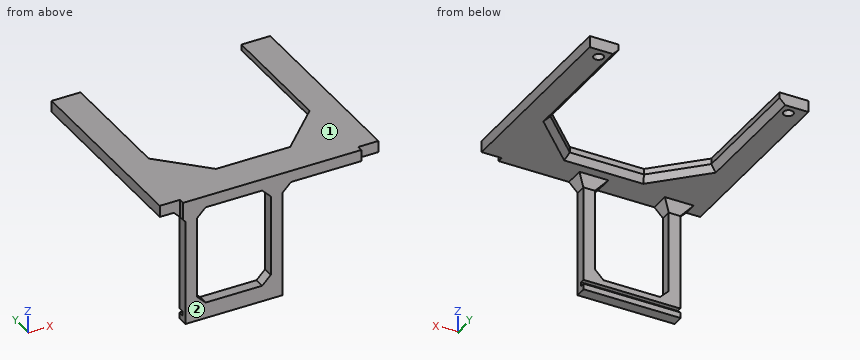
```python
from build123d import *

# Parameters (mm, degrees)
SKETCH6_W           = 33.56421262
SKETCH6_H           = 1.838759269
BOSS_EXTRUDE3_DEPTH = 2
SKETCH7_W           = 33.56421262
SKETCH7_H           = 5.55
BOSS_EXTRUDE4_DEPTH = 2
SKETCH8_W           = 2
SKETCH8_H           = 1.6
BOSS_EXTRUDE5_DEPTH = 33.56421262
SKETCH9_W           = 4
SKETCH9_H           = 3.6
BOSS_EXTRUDE6_DEPTH = 38.203681183
BOSS_EXTRUDE7_DEPTH = 4
CHAMFER2_SIZE       = 3
CHAMFER5_SIZE       = 15
SKETCH11_R          = 1.7
CUT_EXTRUDE1_DEPTH  = 3
CHAMFER7_SIZE       = 2


with BuildPart() as part:
    # Sketch6 → Boss-Extrude3 (new body)
    with BuildSketch(Plane(origin=(0, 0, -103.809020593), x_dir=(-1, 0, 0), z_dir=(0, 0, -1))):
        with Locations((54.699348296, -69.800699844)):
            Rectangle(SKETCH6_W, SKETCH6_H)
    extrude(amount=BOSS_EXTRUDE3_DEPTH)

    # Sketch7 → Boss-Extrude4 (add)
    with BuildSketch(Plane.XZ.offset(70.720079478)):
        with Locations((-54.699348296, -103.034020593)):
            Rectangle(SKETCH7_W, SKETCH7_H)
    extrude(amount=BOSS_EXTRUDE4_DEPTH)

    # Sketch8 → Boss-Extrude5 (add)
    with BuildSketch(Plane(origin=(-37.917241986, 0, 0), x_dir=(0, 0, -1), z_dir=(1, 0, 0))):
        with Locations((101.259020593, -69.920079478)):
            Rectangle(SKETCH8_W, SKETCH8_H)
    extrude(amount=-BOSS_EXTRUDE5_DEPTH)

    # Sketch9 → Boss-Extrude6 (add)
    with BuildSketch(Plane.XY.offset(-100.259020593)):
        with Locations((-69.481454606, -70.920079478)):
            Rectangle(SKETCH9_W, SKETCH9_H)
        with Locations((-39.917241986, -70.920079478)):
            Rectangle(SKETCH9_W, SKETCH9_H)
    extrude(amount=BOSS_EXTRUDE6_DEPTH)

    # Sketch10 → Boss-Extrude7 (add)
    with BuildSketch(Plane.XY.offset(-62.055339411)):
        Polygon((-79.3, -70.770079478), (-72.25, -70.770079478), (-72.25, -72.720079478), (-71.481454606, -72.720079478), (-71.481454606, -69.120079478), (-67.481454606, -69.120079478), (-67.481454606, -72.720079478), (-41.917241986, -72.720079478), (-41.917241986, -69.120079478), (-37.917241986, -69.120079478), (-37.917241986, -72.720079478), (-10.55, -72.720079478), (-10.55, -70.770079478), (-3.6, -70.770079478), (-3.6, -3.05), (-13.6, -3.05), (-13.600000688, -60.770079478), (-69.3, -60.770079478), (-69.3, -3.05), (-79.3, -3.05), align=None)
    extrude(amount=-BOSS_EXTRUDE7_DEPTH)

    # Chamfer2
    chamfer2_edges = [part.edges().sort_by_distance(p)[0] for p in [
        (-41.917241986, -70.920079478, -100.259020593),
        (-67.481454606, -70.920079478, -100.259020593),
        (-41.917241986, -70.920079478, -66.055339411),
        (-39.917241986, -69.120079478, -66.055339411),
        (-37.917241986, -70.920079478, -66.055339411),
        (-67.481454606, -70.920079478, -66.055339411),
        (-69.481454606, -69.120079478, -66.055339411),
        (-71.481454606, -70.920079478, -66.055339411),
    ]]
    chamfer(chamfer2_edges, length=CHAMFER2_SIZE)

    # Chamfer5
    chamfer5_edges = [part.edges().sort_by_distance(p)[0] for p in [
        (-69.3, -60.770079478, -64.055339411),
        (-13.600000688, -60.770079478, -64.055339411),
    ]]
    chamfer(chamfer5_edges, length=CHAMFER5_SIZE)

    # Sketch11 → Cut-Extrude1 (cut)
    with BuildSketch(Plane(origin=(0, 0, -66.055339411), x_dir=(-1, 0, 0), z_dir=(0, 0, -1))):
        with Locations((8.6, -6.55)):
            Circle(SKETCH11_R)
        with Locations((74.3, -6.55)):
            Circle(SKETCH11_R)
    extrude(amount=-CUT_EXTRUDE1_DEPTH, mode=Mode.SUBTRACT)

    # Chamfer7
    chamfer7_edges = [part.edges().sort_by_distance(p)[0] for p in [
        (-41.450000344, -60.770079478, -66.055339411),
        (-21.100000599, -53.270079478, -66.055339411),
        (-61.8, -53.270079478, -66.055339411),
        (-69.3, -24.410039739, -66.055339411),
        (-13.600000255, -24.410039739, -66.055339411),
    ]]
    chamfer(chamfer7_edges, length=CHAMFER7_SIZE)


solid = part.part
```
Source: CAD feature listing. Evaluate the final solid. Frame: model axes, mm. Face numbers are marked on the shaded views. Round coordinates to 2 decimals unless told otherwise and drop trailing zeros. Loops run counter-clockwise (first coordinate to the right, second up) from the corner with the lowest first, then second, coordinate; pieces in that order, holes last. Notation, with made-up numbers: M -39.5,1.25 L 14.5,1.25 A3 ccw 14.5,6.25 Z; hole C 65,-22.5 d8. An arc over 180 degrees is marked long. Use a Markdown table: item, result. Add a question column.
1. Pull-direction query (Z, two-part tool) for the marked faces 1 and 2; classes: +Z half, -Z half, draft (parallel to the pull), parting line (faces both ways), or undercut.
2. Cut plane B-B, the plane y = -6.55. Output: boundary loops of the cut face in (x, z).
3. Cut plane A-A, the plane z = -89. Output: boundary loops of the cut face in (x, y).
4. Cut plane C-C, the plane x = -63.5. Output: boundary loops of the cut face in (y, z).
5. Ray query, line 1 along Y through (x, z) = (-74.3, -65.15); line 2 along X through (y, z) = (-6, -64); line 3 along X through (y, z) = (-6, -63). Return the intervals inside material, ascending. Write a range as [from, to].
6. Cut plane D-D, the plane x = -8.6. Output: boundary loops of the cut face in (y, z).
7. Contact query for flat-ended pins moving along their axis: pin 1 (1 mm diameter, centred on x = -38.5, z = -63, fed in from +Y); pin 2 (1.1 mm diameter, centred on y = -71, z = -83.5, fed in from -X); pin 3 (1.5 mm diameter, centred on x = -67.5, y = -17.5, fed in from -Z); pin 4 (1.1 mm diameter, centred on y = -70.5, z = -81.5, fed in from +X). Output: stop coordinate, or through.
Solution:
| question | item | result |
|---|---|---|
| 1 | face 1 | +Z half |
| 1 | face 2 | draft |
| 2 | outline | M -79.3,-66.06 L -76,-66.06 L -76,-63.06 L -72.6,-63.06 L -72.6,-66.06 L -71.3,-66.06 L -69.3,-64.06 L -69.3,-62.06 L -79.3,-62.06 Z; M -13.6,-64.06 L -11.6,-66.06 L -10.3,-66.06 L -10.3,-63.06 L -6.9,-63.06 L -6.9,-66.06 L -3.6,-66.06 L -3.6,-62.06 L -13.6,-62.06 Z |
| 3 | outline | M -71.48,-72.72 L -67.48,-72.72 L -67.48,-69.12 L -71.48,-69.12 Z; M -41.92,-72.72 L -37.92,-72.72 L -37.92,-69.12 L -41.92,-69.12 Z |
| 4 | outline | M -72.72,-105.81 L -68.88,-105.81 L -68.88,-103.81 L -70.72,-103.81 L -70.72,-102.26 L -69.12,-102.26 L -69.12,-100.26 L -72.72,-100.26 Z; M -72.72,-66.06 L -54.4,-66.06 L -51.57,-64.06 L -51.57,-62.06 L -72.72,-62.06 Z |
| 5 | line 1 | y = [-70.77, -8.25], [-4.85, -3.05] |
| 5 | line 2 | x = [-79.3, -75.91], [-72.69, -69.3], [-13.6, -10.21], [-6.99, -3.6] |
| 5 | line 3 | x = [-79.3, -69.3], [-13.6, -3.6] |
| 6 | outline | M -70.77,-66.06 L -8.25,-66.06 L -8.25,-63.06 L -4.85,-63.06 L -4.85,-66.06 L -3.05,-66.06 L -3.05,-62.06 L -70.77,-62.06 Z |
| 7 | pin 1 | stops at y = -60.77 |
| 7 | pin 2 | stops at x = -71.48 |
| 7 | pin 3 | passes through |
| 7 | pin 4 | stops at x = -37.92 |
